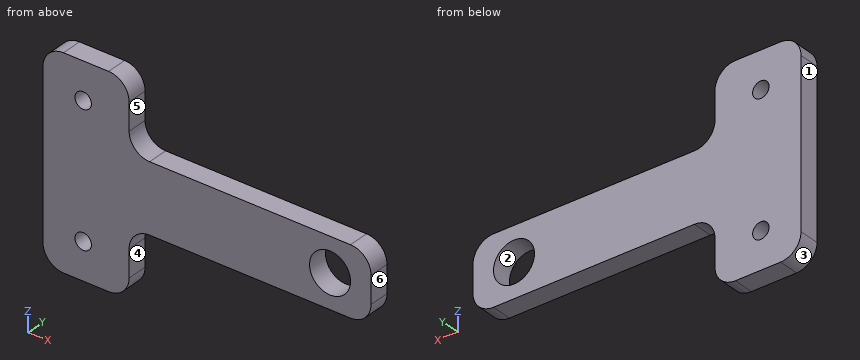
from build123d import *

# Parameters (mm, degrees)
SKETCH1_W           = 29.5
SKETCH1_H           = 8.333333334
SKETCH1_R           = 2.5
SKETCH1_R_2         = 1
BOSS_EXTRUDE1_DEPTH = 2.5
FILLET1_R           = 2.5


with BuildPart() as part:
    # Sketch1 → Boss-Extrude1 (new body)
    with BuildSketch(Plane(origin=(0, 0, 0), x_dir=(1, 0, 0), z_dir=(0, 1, 0))):
        with Locations((25.25, 12.5)):
            Rectangle(SKETCH1_W, SKETCH1_H)
        with Locations((35, 12.5)):
            Circle(SKETCH1_R, mode=Mode.SUBTRACT)
        Polygon((10.5, 25), (1.052631579, 25), (0, 25), (0, 0), (10.5, 0), (10.5, 8.333333333), (10.5, 16.666666667), align=None)
        with Locations((4.9, 4.5)):
            Circle(SKETCH1_R_2, mode=Mode.SUBTRACT)
        with Locations((4.9, 20.5)):
            Circle(SKETCH1_R_2, mode=Mode.SUBTRACT)
    extrude(amount=BOSS_EXTRUDE1_DEPTH)

    # Fillet1
    fillet1_edges = [part.edges().sort_by_distance(p)[0] for p in [
        (40, 1.25, -8.333333333),
        (10.5, 1.25, -8.333333333),
        (10.5, 1.25, 0),
        (0, 1.25, 0),
        (0, 1.25, -25),
        (10.5, 1.25, -25),
        (10.5, 1.25, -16.666666667),
        (40, 1.25, -16.666666667),
    ]]
    fillet(fillet1_edges, radius=FILLET1_R)


solid = part.part
Verification items for the finished model (mm, model axes). Face numbers are marked on the shaded views. A direction names the side the tool comes from. Give positions to 0.01 mm unless a question says otherwise; leave off trailing zeros. Loops run counter-clockwise (first coordinate to the right, second up) from the corner with the lowest first, then second, coordinate; pieces in that order, holes last. Notation, with made-up numbers: (61, -22.5) - (76, -22.5) arc R14 ccw to (76, -16.5) - close; hole circle Ø10 at (77.5, 17). An arc over 180 degrees is marked (long way). Write item = value, one per line. Start each with the question number.
Q1. Cross-section at A-A, the plane z = -12.5. Enter the section's corners in (x, y), and give its area (3 significant figures).
Q2. Cross-section at B-B, the plane y = 0.6. Enter the section's corners in (x, z), and give its area (3 significant figures).
Q3. Mould release check, pull along Z, two halves, no side actions. Record for the marked faces 1, 2 and 3: released by +Z, released by -Z, zero draft, split by the parting line, or undercut.
Q4. Cross-section at C-C, the plane x = 4.9. Enter the section's corners in (y, z).
Q5. Cross-section at D-D, the plane z = -4.5. Enter the section's corners in (x, y).
Q6. Tool access check on the marked faces 4, 5 and 6. Record the directions out of +Z, -Z, +X, -X, +Y, -Y that give a thin tool (end or side, any length) a straight path to the whole face; none if there is none.
Q7. Depth check by flat-ended pin: P1, Ø0.8, axis at y = 1.5, z = -3.5, coming from the +X side; P2, Ø1.8, axis at x = 4.9, z = -20.5, coming from the -Y side; P3, Ø1.5, axis at x = 15, y = 1.5, coming from the -Z side; P4, Ø3, axis at x = 4.9, z = -4.5, coming from the -Y side. Enter the tip coordinate at first touch or a pass-through.
Q8. Thickness scan on line 1 (Z direction, x = 4.9, y = 0.9); line 2 (Z direction, x = 35, y = 1.3); line 3 (X direction, y = 1.95, z = -4.5). Record the ranges inside material, lowest first.
Answer key:
q1.outline = (0, 0) - (32.5, 0) - (32.5, 2.5) - (0, 2.5) - close; (37.5, 0) - (40, 0) - (40, 2.5) - (37.5, 2.5) - close
q1.area = 87.5 mm^2
q2.outline = (0, -22.5) arc R2.5 ccw to (2.5, -25) - (8, -25) arc R2.5 ccw to (10.5, -22.5) - (10.5, -19.17) arc R2.5 cw to (13, -16.67) - (37.5, -16.67) arc R2.5 ccw to (40, -14.17) - (40, -10.83) arc R2.5 ccw to (37.5, -8.33) - (13, -8.33) arc R2.5 cw to (10.5, -5.83) - (10.5, -2.5) arc R2.5 ccw to (8, 0) - (2.5, 0) arc R2.5 ccw to (0, -2.5) - close; hole circle Ø2 at (4.9, -20.5); hole circle Ø2 at (4.9, -4.5); hole circle Ø5 at (35, -12.5)
q2.area = 477 mm^2
q3.face_1 = zero draft
q3.face_2 = undercut
q3.face_3 = released by -Z
q4.outline = (0, -25) - (2.5, -25) - (2.5, -21.5) - (0, -21.5) - close; (0, -19.5) - (2.5, -19.5) - (2.5, -5.5) - (0, -5.5) - close; (0, -3.5) - (2.5, -3.5) - (2.5, 0) - (0, 0) - close
q5.outline = (0, 0) - (3.9, 0) - (3.9, 2.5) - (0, 2.5) - close; (5.9, 0) - (10.5, 0) - (10.5, 2.5) - (5.9, 2.5) - close
q6.face_4 = -Z, +X, +Y, -Y
q6.face_5 = +Z, +X, +Y, -Y
q6.face_6 = +Z, -Z, +X, +Y, -Y
q7.P1 = 10.5
q7.P2 = through
q7.P3 = -16.67
q7.P4 = 0
q8.line_1 = -25 to -21.5, -19.5 to -5.5, -3.5 to 0
q8.line_2 = -16.67 to -15, -10 to -8.33
q8.line_3 = 0 to 3.9, 5.9 to 10.5
